Autodesk Inventor part; units mm, degrees
ref_plane "YZ Plane" through (0, 0, 0) normal (1, 0, 0) x (0, 1, 0)
ref_plane "XZ Plane" through (0, 0, 0) normal (0, 1, 0) x (-1, 0, 0)
ref_plane "XY Plane" through (0, 0, 0) normal (0, 0, 1) x (1, 0, 0)
sketch "Sketch1" plane through (0, 0, 0) normal (0, 0, 1) x (1, 0, 0)
  circle A0 centre (0, 0) radius 23.8125
  dimension "d0" = 47.625
extrude "Extrusion1" add sketch "Sketch1" along normal blind 25.4
sketch "Sketch2" plane through (0, 0, 25.4) normal (0, 0, 1) x (1, 0, 0)
  circle A0 centre (0, 0) radius 23.8125
  circle A1 centre (0, 0) radius 11.1125
  dimension "d3" = 22.225
extrude "Extrusion2" add sketch "Sketch2" along normal blind 0.7937 contours A1
sketch "Sketch3" plane through (0, 0, 26.1938) normal (0, 0, 1) x (1, 0, 0)
  circle A0 centre (0, 0) radius 11.1125
  circle A1 centre (0, 0) radius 7.9375
  dimension "d6" = 15.875
extrude "Extrusion3" cut sketch "Sketch3" against normal through all contours A1
sketch "Sketch4" plane through (0, 0, 0) normal (0, 1, 0) x (-1, 0, 0)
  line L0 (7.9375, 0) -> (-7.9375, 0)
  line L1 (-7.9375, 26.1938) -> (7.9375, 26.1938)
  circle A0 centre (0, 12.7) radius 3.175
  line L2 (0, 0) -> (0, 26.1938)
  line L3 (23.8125, 25.4) -> (-23.8125, 25.4)
  dimension "d9" = 6.35
  dimension "d10" = 12.7
extrude "Extrusion4" cut sketch "Sketch4" along normal through all both and the other way through all
mirror "Mirror1" about plane through (0, 0, 0) normal (0, 0, -1)
properties part number "Winch Body"
Can you work these out from the model? Positions are in its coordinate system, mm. A direction names the side the tool comes from. Round coordinates to 2 decimals unless told otherwise and drop trailing zeros. Loops run counter-clockwise (first coordinate to the right, second up) from the corner with the lowest first, then second, coordinate; pieces in that order, holes last. Notation, with made-up numbers: (-13.5, 21.5) - (34.5, 21.5) arc R7 ccw to (34.5, 27.5) - close; hole circle Ø4 at (-4, -1). An arc over 180 degrees is marked (long way). Answer in a Markdown table with one row per item. Add a question column.
Q1. I want a section at D-D on x = 6.5. List the corners of the cut face in (y, z) for me, and give its area (3 significant figures).
Q2. We'd pull the mould along Z, two halves only. Please class faces 4 (the flat face through (-10.2, -5, -25.4)), 5 (the flat face through (-8, 3, 26.194)), 6 (the cylindrical face through (0.69, -15.43, -15.8)), 7 (the cylindrical face through (10.6, -3.34, 25.79)): pulls with the +Z half, pulls with the -Z half, needs draft (parallel to the pull), parting line crosses it, or undercut.
Q3. I want a section at B-B on x = 1.5. Count the separate pieces of the cut face and the enclosed holes in it, and give its area (3 significant figures).
Q4. Which directions (+Z, -Z, +X, -X, +Y, -Y) give clear straight access to the entire face, cutting with the end or side of a thin tool? Please do faces 1 (the cylindrical face through (0.69, 15.66, -15.8)), 2 (the cylindrical face through (10.6, 3.34, -25.79)), 3 (the flat face through (10.2, -5, 25.4)).
Q5. I want a section at A-A on y = 0. List the corners of the cut face in (x, z) for me.
Q6. I want a section at C-C on z = 12.7. List the corners of the cut face in (x, y) for me (1 decimal).
Q7. For pin 1 Ø10 at (x, z) = (-9, -10.5) entering from +Y; pin 2 Ø10 at (y, z) = (-14.5, 10.5) entering from +X; pin 3 Ø7.5 at (x, z) = (0, -12.7) entering from +Y; pin 4 Ø8 at (y, z) = (-16.5, 4.5) entering from +X, each with a flat end and sliding along its axis, tell me the tip position at first contact or that it passes through.
Q8. I need wall thicknesses on L1, parallel to Z at x = 0, y = 17 (3 decimals); L2, parallel to Z at x = 0, y = 11 (3 decimals); L3, parallel to X at y = -17.75, z = 12.7 (3 decimals). Which ranges of each line are inside material? Lowest first, please.
A:
| question | item | result |
|---|---|---|
| 1 | outline | (-22.91, -25.4) - (-9.01, -25.4) - (-9.01, -26.19) - (-4.56, -26.19) - (-4.56, 26.19) - (-9.01, 26.19) - (-9.01, 25.4) - (-22.91, 25.4) - close; (4.56, -26.19) - (9.01, -26.19) - (9.01, -25.4) - (22.91, -25.4) - (22.91, 25.4) - (9.01, 25.4) - (9.01, 26.19) - (4.56, 26.19) - close |
| 1 | area | 1,880 mm^2 |
| 2 | face 4 | pulls with the -Z half |
| 2 | face 5 | pulls with the +Z half |
| 2 | face 6 | undercut |
| 2 | face 7 | needs draft |
| 3 | separate pieces | 6 |
| 3 | enclosed holes | 0 |
| 3 | area | 1,280 mm^2 |
| 4 | face 1 | +Y, -Y |
| 4 | face 2 | -Z |
| 4 | face 3 | +Z |
| 5 | outline | (-23.81, -25.4) - (-11.11, -25.4) - (-11.11, -26.19) - (-7.94, -26.19) - (-7.94, 26.19) - (-11.11, 26.19) - (-11.11, 25.4) - (-23.81, 25.4) - close; (7.94, -26.19) - (11.11, -26.19) - (11.11, -25.4) - (23.81, -25.4) - (23.81, 25.4) - (11.11, 25.4) - (11.11, 26.19) - (7.94, 26.19) - close |
| 6 | outline | (-3.2, -23.6) - (-3.2, -7.3) arc R7.9 cw to (-3.2, 7.3) - (-3.2, 23.6) arc R23.8 ccw to start; (3.2, -23.6) arc R23.8 ccw to (3.2, 23.6) - (3.2, 7.3) arc R7.9 cw to (3.2, -7.3) - close |
| 7 | pin 1 | y = 23.47 |
| 7 | pin 2 | x = 21.84 |
| 7 | pin 3 | y = 23.81 |
| 7 | pin 4 | x = 20.27 |
| 8 | L1 | -25.4 to -15.875, -9.525 to 9.525, 15.875 to 25.4 |
| 8 | L2 | -26.194 to -15.875, -9.525 to 9.525, 15.875 to 26.194 |
| 8 | L3 | -15.874 to -3.175, 3.175 to 15.874 |
